```python
from build123d import *

# Parameters (mm, degrees)
F0_W     = 120
F0_H     = 350
F1_DEPTH = 60
F2_W     = 50
F2_H     = 300
F3_DEPTH = 30
F4_T     = -2.5
F5_W     = 120
F5_H     = 3
F6_DEPTH = 25
F8_DEPTH = 25


with BuildPart() as f1:
    # F0 (on Front) → F1 (new body)
    with BuildSketch(Plane.XZ):
        with Locations((60, 175)):
            Rectangle(F0_W, F0_H)
    extrude(amount=F1_DEPTH)

    # F2 (on face) → F3 (cut)
    with BuildSketch(Plane.XZ.offset(60)):
        with Locations((95, 170)):
            Rectangle(F2_W, F2_H)
    extrude(amount=-F3_DEPTH, mode=Mode.SUBTRACT)

    # F4
    f4_openings = [f1.faces().sort_by_distance(p)[0] for p in [
        (95, -45, 20),
        (70, -45, 170),
        (95, -30, 170),
        (95, -45, 320),
    ]]
    offset(amount=F4_T, openings=f4_openings)

    # F5 (on face) → F6 (join)
    with BuildSketch(Plane.XY.offset(350)):
        with Locations((60, -1.5)):
            Rectangle(F5_W, F5_H)
    extrude(amount=F6_DEPTH)

    # F7 (on face) → F8 (cut)
    with BuildSketch(Plane.XZ.offset(3)):
        with BuildLine():
            ThreePointArc((64.953983, 364.60001), (63.505749, 368.119237), (60, 369.599798))
            ThreePointArc((60, 369.599798), (56.434756, 368.151776), (54.953983, 364.60001))
            Line((54.953983, 364.60001), (44.953983, 364.60001))
            ThreePointArc((44.953983, 364.60001), (41.203983, 360.85001), (44.953983, 357.10001))
            Line((44.953983, 357.10001), (74.953983, 357.10001))
            ThreePointArc((74.953983, 357.10001), (78.703983, 360.85001), (74.953983, 364.60001))
            Line((74.953983, 364.60001), (64.953983, 364.60001))
        make_face()
    extrude(amount=-F8_DEPTH, mode=Mode.SUBTRACT)


solid = f1.part
```
CAD build for the part. Positions are in the model's coordinates, mm. A direction names the side the tool comes from. Give positions to 0.01 mm unless a question says otherwise; leave off trailing zeros. Loops run counter-clockwise (first coordinate to the right, second up) from the corner with the lowest first, then second, coordinate; pieces in that order, holes last. Notation, with made-up numbers: (69, -7.75) -> (114, -7.75) arc R20 cw to (114, 28.25) -> close; hole circle Ø4 at (-22, 59.25). An arc over 180 degrees is marked (long way). Use a Markdown table: item, result.
1. Wall check: L1, parallel to Z at x = 17, y = -11; L2, parallel to X at y = -6, z = 304; L3, parallel to Y at x = 28, z = 97. Give the ranges that are in metal, low to high. Write a range as [from, to].
Check result:
| item | result |
|---|---|
| L1 | z = [0, 2.5], [347.5, 350] |
| L2 | x = [0, 2.5], [117.5, 120] |
| L3 | y = [-60, -57.5], [-2.5, 0] |
2. Slice it at B-B (y = -20). List the corners of the cut face in (x, z).
Check result:
| item | result |
|---|---|
| outline | (0, 0) -> (120, 0) -> (120, 350) -> (0, 350) -> close; hole (2.5, 2.5) -> (117.5, 2.5) -> (117.5, 347.5) -> (2.5, 347.5) -> close |
3. Slice it at A-A (x = 23). List the corners of the cut face in (y, z).
Check result:
| item | result |
|---|---|
| outline | (-60, 0) -> (0, 0) -> (0, 375) -> (-3, 375) -> (-3, 350) -> (-60, 350) -> close; hole (-57.5, 2.5) -> (-2.5, 2.5) -> (-2.5, 347.5) -> (-57.5, 347.5) -> close |
4. Slice it at C-C (z = 50.5). List the corners of the cut face in (x, y), plus the area to 3 significant figures.
Check result:
| item | result |
|---|---|
| outline | (0, -60) -> (70, -60) -> (70, -57.5) -> (2.5, -57.5) -> (2.5, -2.5) -> (117.5, -2.5) -> (117.5, -30) -> (120, -30) -> (120, 0) -> (0, 0) -> close |
| area | 681 mm^2 |
5. Slice it at D-D (y = -50.5). List the corners of the cut face in (x, z), plus the area to 4 significant figures.
Check result:
| item | result |
|---|---|
| outline | (0, 0) -> (120, 0) -> (120, 20) -> (117.5, 20) -> (117.5, 2.5) -> (2.5, 2.5) -> (2.5, 347.5) -> (117.5, 347.5) -> (117.5, 320) -> (120, 320) -> (120, 350) -> (0, 350) -> close |
| area | 1,575 mm^2 |
6. Flat gauge pins, fed straight in: pin 1 (12.5 mm diameter, centred on x = 57.5, z = 361, fed in from -Y); pin 2 (3 mm diameter, centred on y = -58.5, z = 184, fed in from +X); pin 3 (15 mm diameter, centred on x = 91, y = -51, fed in from +Z). Where does each tip first touch, or does it go through?
Check result:
| item | result |
|---|---|
| pin 1 | stops at y = -3 |
| pin 2 | stops at x = 70 |
| pin 3 | stops at z = 350 |
7. Which spindle directions (+Z, -Z, +X, -X, +Y, -Y) get a long thin tool onto all of the face, cutting with end or side? Do faces 5 (the flat face through (59.2, -3, 356.8)), 6 (the flat face through (102, -58, 20)), 7 (the flat face through (117.5, -24, 173)). Say none if no direction does.
Check result:
| item | result |
|---|---|
| face 5 | +Z, +X, -X, -Y |
| face 6 | +X, -Y |
| face 7 | none |
8. Mould opens along X. For faces 1 (the flat face through (59, -30, 347.5)), 2 (the flat face through (59, 0, 185)), 3 (the flat face through (0, -30, 143)), 4 (the flat face through (2.5, -30, 173)) say: pulls with the +X half, pulls with the -X half, needs draft (parallel to the pull), parting line crosses it, or undercut.
Check result:
| item | result |
|---|---|
| face 1 | undercut |
| face 2 | needs draft |
| face 3 | pulls with the -X half |
| face 4 | undercut |
